Input: part model. Units: mm. Frame: model coordinates. A direction names the side the tool comes from. Round coordinates to 2 decimals unless told otherwise and drop trailing zeros. Write each loop counter-clockwise with the first axis right and the second up, starting at its lowest first coordinate (ties: lowest second). Pieces come first, ordered by that corner, then holes. Notation, with made-up numbers: (45.25, 14) - (69.25, 14) arc R5 ccw to (69.25, 21) - close; hole circle Ø6 at (-18.5, 83). An arc over 180 degrees is marked (long way). One line per item, written item: value. Start each with the question number.
```python
from build123d import *

# Parameters (mm, degrees)
BOSS_EXTRUDE1_DEPTH     = 3
SKETCH5_W               = 3
SKETCH5_H               = 30
CUT_EXTRUDE3_DEPTH      = 3
SKETCH7_R               = 7
CUT_EXTRUDE4_DEPTH      = 3
CUT_EXTRUDE6_DEPTH      = 1
CUT_EXTRUDE6_DEPTH_BACK = 3


with BuildPart() as part:
    # Sketch1 → Boss-Extrude1 (new body)
    with BuildSketch(Plane.XY):
        with BuildLine():
            Line((-55, -71.239034244), (-35.5, -71.239034244))
            Line((-35.5, -71.239034244), (-35, -64.236863152))
            Line((-35, -64.236863152), (-34.5, -64.236863152))
            Line((-34.5, -64.236863152), (-34.5, -73.236863152))
            Line((-34.5, -73.236863152), (-35, -74.236863152))
            Line((-35, -74.236863152), (-35.5, -74.736863152))
            Line((-35.5, -74.736863152), (-35.5, -75.736863152))
            Line((-35.5, -75.736863152), (-34, -77.236863152))
            Line((-34, -77.236863152), (-32.5, -77.236863152))
            Line((-32.5, -77.236863152), (-32, -64.236863152))
            Line((-32, -64.236863152), (-31.5, -64.236863152))
            Line((-31.5, -64.236863152), (-31.5, -77.236863152))
            Line((-31.5, -77.236863152), (-23.5, -77.236863152))
            Line((-23.5, -77.236863152), (-23.5, -64.236863152))
            Line((-23.5, -64.236863152), (-23, -64.236863152))
            Line((-23, -64.236863152), (-22.5, -77.236863152))
            Line((-22.5, -77.236863152), (-21, -77.236863152))
            Line((-21, -77.236863152), (-19.5, -75.736863152))
            Line((-19.5, -75.736863152), (-19.5, -74.736863152))
            Line((-19.5, -74.736863152), (-20, -74.236863152))
            Line((-20, -74.236863152), (-20.5, -73.236863152))
            Line((-20.5, -73.236863152), (-20.5, -64.236863152))
            Line((-20.5, -64.236863152), (-20, -64.236863152))
            Line((-20, -64.236863152), (-19.5, -71.239034244))
            Line((-19.5, -71.239034244), (19.5, -71.239034244))
            Line((19.5, -71.239034244), (20, -64.236863152))
            Line((20, -64.236863152), (20.5, -64.236863152))
            Line((20.5, -64.236863152), (20.5, -73.236863152))
            Line((20.5, -73.236863152), (20, -74.236863152))
            Line((20, -74.236863152), (19.5, -74.736863152))
            Line((19.5, -74.736863152), (19.5, -75.736863152))
            Line((19.5, -75.736863152), (21, -77.236863152))
            Line((21, -77.236863152), (22.5, -77.236863152))
            Line((22.5, -77.236863152), (23, -64.236863152))
            Line((23, -64.236863152), (23.5, -64.236863152))
            Line((23.5, -64.236863152), (23.5, -77.236863152))
            Line((23.5, -77.236863152), (31.5, -77.236863152))
            Line((31.5, -77.236863152), (31.5, -64.236863152))
            Line((31.5, -64.236863152), (32, -64.236863152))
            Line((32, -64.236863152), (32.5, -77.236863152))
            Line((32.5, -77.236863152), (34, -77.236863152))
            Line((34, -77.236863152), (35.5, -75.736863152))
            Line((35.5, -75.736863152), (35.5, -74.736863152))
            Line((35.5, -74.736863152), (35, -74.236863152))
            Line((35, -74.236863152), (34.5, -73.236863152))
            Line((34.5, -73.236863152), (34.5, -64.236863152))
            Line((34.5, -64.236863152), (35, -64.236863152))
            Line((35, -64.236863152), (35.5, -71.239034244))
            Line((35.5, -71.239034244), (55, -71.239034244))
            ThreePointArc((55, -71.239034244), (80.777472107, -39.686269666), (90, 0))
            Line((90, 0), (73, 0))
            Line((73, 0), (72.5, -7.002171092))
            Line((72.5, -7.002171092), (72, -7.002171092))
            Line((72, -7.002171092), (72, 1.997828908))
            Line((72, 1.997828908), (72.5, 2.997828908))
            Line((72.5, 2.997828908), (73, 3.497828908))
            Line((73, 3.497828908), (73, 4.497828908))
            Line((73, 4.497828908), (71.5, 5.997828908))
            Line((71.5, 5.997828908), (70, 5.997828908))
            Line((70, 5.997828908), (69.5, -7.002171092))
            Line((69.5, -7.002171092), (69, -7.002171092))
            Line((69, -7.002171092), (69, 5.997828908))
            Line((69, 5.997828908), (61, 5.997828908))
            Line((61, 5.997828908), (61, -7.002171092))
            Line((61, -7.002171092), (60.5, -7.002171092))
            Line((60.5, -7.002171092), (60, 5.997828908))
            Line((60, 5.997828908), (58.5, 5.997828908))
            Line((58.5, 5.997828908), (57, 4.497828908))
            Line((57, 4.497828908), (57, 3.497828908))
            Line((57, 3.497828908), (57.5, 2.997828908))
            Line((57.5, 2.997828908), (58, 1.997828908))
            Line((58, 1.997828908), (58, -7.002171092))
            Line((58, -7.002171092), (57.5, -7.002171092))
            Line((57.5, -7.002171092), (57, 0))
            Line((57, 0), (32, 0))
            Line((32, 0), (32, -4))
            Line((32, -4), (18, -4))
            Line((18, -4), (18, 0))
            Line((18, 0), (-17, 0))
            Line((-17, 0), (-17.5, -7.002171092))
            Line((-17.5, -7.002171092), (-18, -7.002171092))
            Line((-18, -7.002171092), (-18, 1.997828908))
            Line((-18, 1.997828908), (-17.5, 2.997828908))
            Line((-17.5, 2.997828908), (-17, 3.497828908))
            Line((-17, 3.497828908), (-17, 4.497828908))
            Line((-17, 4.497828908), (-18.5, 5.997828908))
            Line((-18.5, 5.997828908), (-20, 5.997828908))
            Line((-20, 5.997828908), (-20.5, -7.002171092))
            Line((-20.5, -7.002171092), (-21, -7.002171092))
            Line((-21, -7.002171092), (-21, 5.997828908))
            Line((-21, 5.997828908), (-29, 5.997828908))
            Line((-29, 5.997828908), (-29, -7.002171092))
            Line((-29, -7.002171092), (-29.5, -7.002171092))
            Line((-29.5, -7.002171092), (-30, 5.997828908))
            Line((-30, 5.997828908), (-31.5, 5.997828908))
            Line((-31.5, 5.997828908), (-33, 4.497828908))
            Line((-33, 4.497828908), (-33, 3.497828908))
            Line((-33, 3.497828908), (-32.5, 2.997828908))
            Line((-32.5, 2.997828908), (-32, 1.997828908))
            Line((-32, 1.997828908), (-32, -7.002171092))
            Line((-32, -7.002171092), (-32.5, -7.002171092))
            Line((-32.5, -7.002171092), (-33, 0))
            Line((-33, 0), (-58, 0))
            Line((-58, 0), (-58, -4))
            Line((-58, -4), (-72, -4))
            Line((-72, -4), (-72, 0))
            Line((-72, 0), (-90, 0))
            ThreePointArc((-90, 0), (-80.777472107, -39.686269666), (-55, -71.239034244))
        make_face()
    extrude(amount=BOSS_EXTRUDE1_DEPTH)

    # Sketch5 → Cut-Extrude3 (cut)
    with BuildSketch(Plane(origin=(0, 0, 0), x_dir=(-1, 0, 0), z_dir=(0, 0, -1))):
        with Locations((-48.5, -27.74)):
            Rectangle(SKETCH5_W, SKETCH5_H)
        with Locations((48.5, -27.74)):
            Rectangle(SKETCH5_W, SKETCH5_H)
    extrude(amount=-CUT_EXTRUDE3_DEPTH, mode=Mode.SUBTRACT)

    # Sketch7 → Cut-Extrude4 (cut)
    with BuildSketch(Plane(origin=(0, 0, 0), x_dir=(-1, 0, 0), z_dir=(0, 0, -1))):
        with Locations((65, -27)):
            Circle(SKETCH7_R)
        with Locations((-65, -27)):
            Circle(SKETCH7_R)
    extrude(amount=-CUT_EXTRUDE4_DEPTH, mode=Mode.SUBTRACT)

    # Sketch8 → Cut-Extrude6 (cut, two sides)
    with BuildSketch(Plane(origin=(0, 0, 0), x_dir=(-1, 0, 0), z_dir=(0, 0, -1))) as cut_extrude6_sk:
        Polygon((-1.5, -320.719998244), (-1.5, -71.239034244), (-1.5, -48.239034244), (1.5, -48.239034244), (1.5, -71.239034244), (1.5, -320.719998244), (1.5, -819.681926243), (-1.5, -819.681926243), align=None)
    extrude(amount=CUT_EXTRUDE6_DEPTH, mode=Mode.SUBTRACT)
    extrude(cut_extrude6_sk.sketch, amount=-CUT_EXTRUDE6_DEPTH_BACK, mode=Mode.SUBTRACT)


solid = part.part
```
Q1. Cut plane B-B, the plane x = 65. Output: boundary loops of the cut face in (y, z).
Q2. Contact query for flat-ended pins moving along their axis: pin 1 Ø0.9 at (y, z) = (-69.5, 2) entering from -X; pin 2 Ø0.8 at (y, z) = (-75, 2) entering from -X; pin 3 Ø1 at (x, z) = (-62, 1.5) entering from +Y. Output: stop coordinate, or through.
Q3. Material intervals for probe 1 along X at (y, z) = (-17, 1.6); probe 2 along Y at (x, z) = (-55, 1.8); probe 3 along X at (y, z) = (-16, 1.25), sorted ascending. Write a range as from..to.
Q4. Cut plane D-D, the plane x = -68.5. Output: boundary loops of the cut face in (y, z).
Q5. Cut plane C-C, the plane z = 1.3. Count the separate pieces of the cut face and the enclosed holes in it, and give its area (3 significant figures).
Q6. Pull-direction query (Y, two-part tool) for faces 1 (the flat face through (-81, 0, 1)), 2 (the flat face through (-48, -42.74, 1)), 3 (the flat face through (-28, -77.237, 1)); classes: pulls with the +Y half, pulls with the -Y half, needs draft (parallel to the pull), parting line crosses it, or undercut.
Q7. Cut plane A-A, the plane y = -27. Output: boundary loops of the cut face in (x, z), and give its area (3 significant figures).
Q8. Access query for faces 4 (the flat face through (-18, -3, 1)), 5 (the flat face through (-45, -71.239, 1)), 6 (the flat face through (22.746, -70.828, 1.479)). Directions: +Z, -Z, +X, -X, +Y, -Y. A direction counts if a zero-diameter tool reaches every point of the face in a straight line with its end or side. Return the directions, or none.
A:
1. outline: (-62.25, 0) - (-34, 0) - (-34, 3) - (-62.25, 3) - close; (-20, 0) - (6, 0) - (6, 3) - (-20, 3) - close
2. pin 1: stops at x = -57.72
2. pin 2: stops at x = -35.5
2. pin 3: stops at y = -4
3. probe 1: x = -88.38..-50, -47..47, 50..88.38
3. probe 2: y = -71.24..0
3. probe 3: x = -88.57..-50, -47..47, 50..88.57
4. outline: (-58.38, 0) - (-33.06, 0) - (-33.06, 3) - (-58.38, 3) - close; (-20.94, 0) - (-4, 0) - (-4, 3) - (-20.94, 3) - close
5. separate pieces: 1
5. enclosed holes: 4
5. area: 10,900 mm²
6. face 1: pulls with the +Y half
6. face 2: undercut
6. face 3: pulls with the -Y half
7. outline: (-85.85, 0) - (-72, 0) - (-72, 3) - (-85.85, 3) - close; (-58, 0) - (-50, 0) - (-50, 3) - (-58, 3) - close; (-47, 0) - (47, 0) - (47, 3) - (-47, 3) - close; (50, 0) - (58, 0) - (58, 3) - (50, 3) - close; (72, 0) - (85.85, 0) - (85.85, 3) - (72, 3) - close
7. area: 413 mm²
8. face 4: +Z, -Z
8. face 5: +Z, -Z, -X, -Y
8. face 6: +Z, -Z, -Y
